Design review of the part built by this model. Coordinates are the model's own, in mm. A direction names the side the tool comes from. Coordinates: 2 decimals unless noted, no trailing zeros. Order: outer loops, then holes, each group sorted by start corner. A loop starts at its lowest first (then second) coordinate and runs counter-clockwise, first axis right, second up. Notation, with made-up numbers: (25.5, 48) -> (77.5, 48) arc R21 ccw to (77.5, 87) -> close; hole circle Ø8 at (40.25, 14). An arc over 180 degrees is marked (long way). Use a Markdown table: item, result. Add a question column.
Q1. Wall thickness on probe 1 along Y at (x, z) = (122, -114.5); probe 2 along Z at (x, y) = (99.5, 3.15); probe 3 along X at (y, z) = (3.2, -123): over which ranges is each line inside the solid? List them lowest first.
Q2. Machinability: for faces 1 (the face through (65, 2, -145)), 2 (the face through (75, 2, -170)), 3 (the face through (84.49, -0.49, -2.85)), 4 (the face through (85, 2, -145)), which of the approach directions +Z, -Z, +X, -X, +Y, -Y give a long, thin tool a straight path to every point of the face, cutting with its end or side? Answer none if there is none.
Q3. Add section B-B (z = -162). State the section outline as (x, y) points, then the cut area to 3 significant figures.
Q4. Add section A-A (y = 2.9). State the section outline as (x, z) points, then the cut area to 3 significant figures.
Q5. Add section C-C (x = 53.5). State the section outline as (y, z) points, then the cut area to 3 significant figures.
Q6. Insertion check: pin 1 (8 mm diameter, centred on x = 57.5, z = -86.5, fed in from -Y); pin 2 (0.8 mm diameter, centred on y = -0.5, z = -110, fed in from +X); pin 3 (2.5 mm diameter, centred on y = 2, z = -139.5, fed in from -X). Each pin has a flat end and moves straight along its axis. Give the tip position at first contact, or say it passes through.
Autodesk Inventor part; units mm, degrees
ref_plane "YZ Plane" through (0, 0, 0) normal (1, 0, 0) x (0, 1, 0)
ref_plane "XZ Plane" through (0, 0, 0) normal (0, 1, 0) x (-1, 0, 0)
ref_plane "XY Plane" through (0, 0, 0) normal (0, 0, 1) x (1, 0, 0)
sketch "Sketch1" plane through (0, 0, 0) normal (0, 1, 0) x (-1, 0, 0)
  line L0 (0, 0) -> (-150, 0)
  line L1 (-150, 0) -> (-150, -120)
  line L2 (0, -120) -> (0, 0)
  line L3 (-65, -120) -> (-85, -120)
  line L4 (-85, -120) -> (-85, -170)
  line L5 (-85, -170) -> (-65, -170)
  line L6 (-65, -170) -> (-65, -120)
  line L7 (-150, -120) -> (-85, -120)
  line L8 (-65, -120) -> (0, -120)
  dimension "d0" = 150
  dimension "d1" = 120
  dimension "d2" = 20
  dimension "d3" = 50
extrude "Extrusion1" add sketch "Sketch1" along normal blind 5
sketch "Sketch2" plane through (0, 0, 0) normal (0, -1, 0) x (1, 0, 0)
  line L0 (0, 0) -> (150, 0)
  line L1 (77.5, 0) -> (72.5, 0)
  line L2 (62.5, -10) -> (62.5, -190)
  line L3 (72.5, -200) -> (77.5, -200)
  line L4 (87.5, -190) -> (87.5, -10)
  arc A0 (62.5, -190) -> (72.5, -200) centre (72.5, -190) ccw
  arc A1 (77.5, -200) -> (87.5, -190) centre (77.5, -190) ccw
  arc A2 (72.5, 0) -> (62.5, -10) centre (72.5, -10) ccw
  arc A3 (87.5, -10) -> (77.5, 0) centre (77.5, -10) ccw
  point P0 (87.5, 0)
  point P1 (62.5, -200)
  point P2 (62.5, 0)
  point P3 (87.5, -200)
  dimension "d6" = 25
  dimension "d7" = 200
  dimension "d8" = 10
extrude "Extrusion2" add sketch "Sketch2" along normal blind 1
properties part number "base"
Established:
| question | item | result |
|---|---|---|
| 1 | probe 1 | 0 to 5 |
| 1 | probe 2 | -120 to 0 |
| 1 | probe 3 | 65 to 85 |
| 2 | face 1 | -Z, -X, +Y |
| 2 | face 2 | -Z, +X, -X, +Y |
| 2 | face 3 | +Z, +X, -Y |
| 2 | face 4 | -Z, +X, +Y |
| 3 | outline | (62.5, -1) -> (87.5, -1) -> (87.5, 0) -> (85, 0) -> (85, 5) -> (65, 5) -> (65, 0) -> (62.5, 0) -> close |
| 3 | area | 125 mm^2 |
| 4 | outline | (0, -120) -> (65, -120) -> (65, -170) -> (85, -170) -> (85, -120) -> (150, -120) -> (150, 0) -> (0, 0) -> close |
| 4 | area | 19,000 mm^2 |
| 5 | outline | (0, -120) -> (5, -120) -> (5, 0) -> (0, 0) -> close |
| 5 | area | 600 mm^2 |
| 6 | pin 1 | y = 0 |
| 6 | pin 2 | x = 87.5 |
| 6 | pin 3 | x = 65 |
